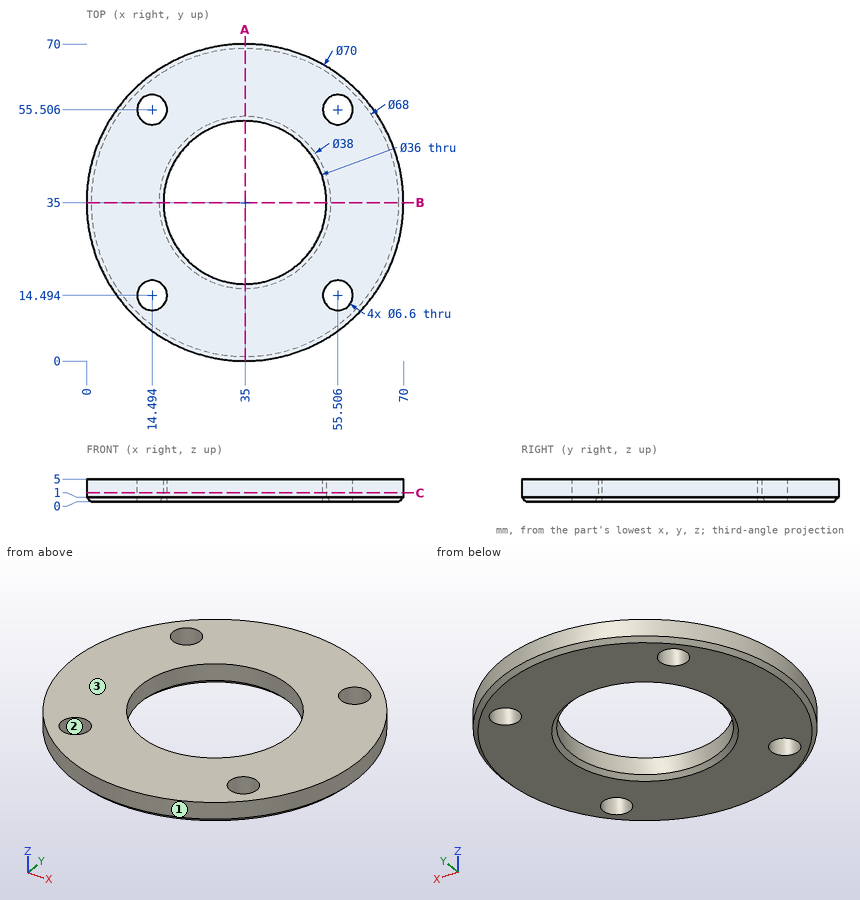
Part print with two shaded views. Sizes in mm from the minimum x, y, z corner. Round coordinates to 2 decimals unless told otherwise and drop trailing zeros. Loops run counter-clockwise (first coordinate to the right, second up) from the corner with the lowest first, then second, coordinate; pieces in that order, holes last. Notation, with made-up numbers: M -23,11.5 L 3,11.5 A12 ccw 3,16.5 Z; hole C -3,-2.5 d10. An arc over 180 degrees is marked long. Return JSON: item names as keys, results as strings. Group by question number.
(1) Mould opens along X. For the marked faces 1, 2 and 3 say: +X half, -X half, draft (parallel to the pull), parting line (faces both ways), or undercut.
(2) Drop flat-ended pins along their axis: P1, Ø4, axis at x = 55.51, y = 14.49, coming from the -Z side; P2, Ø1.5, axis at y = 51, z = 2, coming from the +X side; P3, Ø3, axis at x = 61, y = 9.5, coming from the -Z side; P4, Ø1.5, axis at x = 31, z = 1, coming from the -Y side. Give the stop position or say it passes through.
(3) Wall check: probe 1 along X at (y, z) = (13, 2.65); probe 2 along X at (y, z) = (56, 4.2); probe 3 along Y at (x, z) = (40, 3.65). Give the ranges that are in metal, low to high. Write a range as [from, to].
(4) Saw through at C-C, the plane z = 1.95. List the corners of the cut face in (x, y).
(5) Saw through at A-A, the plane x = 35. List the corners of the cut face in (y, z).
Answer list:
{
 "1": {"face 1": "parting line", "face 2": "undercut", "face 3": "draft"},
 "2": {"P1": "through", "P2": "x = 66.5", "P3": "z = 0.92", "P4": "y = 0.15"},
 "3": {"probe 1": "[7.78, 11.55], [17.44, 52.56], [58.45, 62.22]", "probe 2": "[7, 11.23], [17.76, 52.24], [58.77, 63]", "probe 3": "[0.36, 17.71], [52.29, 69.64]"},
 "4": {"outline": "C 35,35 d70; hole C 14.49,14.49 d6.6; hole C 14.49,55.51 d6.6; hole C 35,35 d36; hole C 55.51,14.49 d6.6; hole C 55.51,55.51 d6.6"},
 "5": {"outline": "M 0,1 L 1,0 L 16,0 L 17,1 L 17,5 L 0,5 Z; M 53,1 L 54,0 L 69,0 L 70,1 L 70,5 L 53,5 Z"}
}
